```python
from build123d import *

# Parameters (mm, degrees)
ESQUISSE1_W             = 54.4
ESQUISSE1_H             = 15
BOSS_EXTRU_1_DEPTH      = 2
ESQUISSE2_W             = 2
ESQUISSE2_H             = 15
BOSS_EXTRU_2_DEPTH      = 35
CONG_1_R                = 1
ENL_V_MAT_EXTRU_1_REACH = 68.403
ESQUISSE3_R             = 1.6
ENL_V_MAT_EXTRU_2_REACH = 69.479
ESQUISSE4_R             = 1.6
ENL_V_MAT_EXTRU_3_REACH = 68.403
ESQUISSE6_R             = 1.5


with BuildPart() as part:
    # Esquisse1 → Boss.-Extru.1 (new body)
    with BuildSketch(Plane(origin=(0, 0, 0), x_dir=(1, 0, 0), z_dir=(0, 1, 0))):
        with Locations((27.2, 7.5)):
            Rectangle(ESQUISSE1_W, ESQUISSE1_H)
    extrude(amount=BOSS_EXTRU_1_DEPTH)

    # Esquisse2 → Boss.-Extru.2 (add)
    with BuildSketch(Plane.XZ):
        with Locations((1, -7.5)):
            Rectangle(ESQUISSE2_W, ESQUISSE2_H)
        with Locations((53.4, -7.5)):
            Rectangle(ESQUISSE2_W, ESQUISSE2_H)
    extrude(amount=BOSS_EXTRU_2_DEPTH)

    # Congé1
    cong_1_edges = [part.edges().sort_by_distance(p)[0] for p in [
        (52.4, 0, -7.5),
        (2, 0, -7.5),
    ]]
    fillet(cong_1_edges, radius=CONG_1_R)

    # Esquisse3 → Enlèv. mat.-Extru.1 (cut, up to next)
    with BuildSketch(Plane(origin=(54.4, 0, 0), x_dir=(0, 0, -1), z_dir=(1, 0, 0)), mode=Mode.PRIVATE) as enl_v_mat_extru_1_sk1:
        with Locations((7.5, -21.65)):
            Circle(ESQUISSE3_R)
    enl_v_mat_extru_1_tool1 = extrude(enl_v_mat_extru_1_sk1.sketch, amount=-ENL_V_MAT_EXTRU_1_REACH, mode=Mode.PRIVATE) & part.part
    add(enl_v_mat_extru_1_tool1.solids().sort_by_distance((54.4, -21.65, -7.5))[0], mode=Mode.SUBTRACT)

    # Esquisse4 → Enlèv. mat.-Extru.2 (cut, up to next)
    with BuildSketch(Plane(origin=(0, 2, 0), x_dir=(1, 0, 0), z_dir=(0, 1, 0)), mode=Mode.PRIVATE) as enl_v_mat_extru_2_sk1:
        with Locations(Location((42.4, 7.5, 0), (0, 0, 270))):
            Circle(ESQUISSE4_R)
    enl_v_mat_extru_2_tool1 = extrude(enl_v_mat_extru_2_sk1.sketch, amount=-ENL_V_MAT_EXTRU_2_REACH, mode=Mode.PRIVATE) & part.part
    # Esquisse4 → Enlèv. mat.-Extru.2 (cut, up to next)
    with BuildSketch(Plane(origin=(0, 2, 0), x_dir=(1, 0, 0), z_dir=(0, 1, 0)), mode=Mode.PRIVATE) as enl_v_mat_extru_2_sk2:
        with Locations(Location((6.4, 7.5, 0), (0, 0, 270))):
            Circle(ESQUISSE4_R)
    enl_v_mat_extru_2_tool2 = extrude(enl_v_mat_extru_2_sk2.sketch, amount=-ENL_V_MAT_EXTRU_2_REACH, mode=Mode.PRIVATE) & part.part
    # Esquisse4 → Enlèv. mat.-Extru.2 (cut, up to next)
    with BuildSketch(Plane(origin=(0, 2, 0), x_dir=(1, 0, 0), z_dir=(0, 1, 0)), mode=Mode.PRIVATE) as enl_v_mat_extru_2_sk3:
        with Locations(Location((24.4, 7.5, 0), (0, 0, 270))):
            Circle(ESQUISSE4_R)
    enl_v_mat_extru_2_tool3 = extrude(enl_v_mat_extru_2_sk3.sketch, amount=-ENL_V_MAT_EXTRU_2_REACH, mode=Mode.PRIVATE) & part.part
    add(enl_v_mat_extru_2_tool1.solids().sort_by_distance((42.4, 2, -7.5))[0], mode=Mode.SUBTRACT)
    add(enl_v_mat_extru_2_tool2.solids().sort_by_distance((6.4, 2, -7.5))[0], mode=Mode.SUBTRACT)
    add(enl_v_mat_extru_2_tool3.solids().sort_by_distance((24.4, 2, -7.5))[0], mode=Mode.SUBTRACT)

    # Esquisse6 → Enlèv. mat.-Extru.3 (cut, up to next)
    with BuildSketch(Plane.ZY, mode=Mode.PRIVATE) as enl_v_mat_extru_3_sk1:
        with Locations((-7.5, -13.86)):
            Circle(ESQUISSE6_R)
    enl_v_mat_extru_3_tool1 = extrude(enl_v_mat_extru_3_sk1.sketch, amount=-ENL_V_MAT_EXTRU_3_REACH, mode=Mode.PRIVATE) & part.part
    # Esquisse6 → Enlèv. mat.-Extru.3 (cut, up to next)
    with BuildSketch(Plane.ZY, mode=Mode.PRIVATE) as enl_v_mat_extru_3_sk2:
        with Locations((-7.5, -29.86)):
            Circle(ESQUISSE6_R)
    enl_v_mat_extru_3_tool2 = extrude(enl_v_mat_extru_3_sk2.sketch, amount=-ENL_V_MAT_EXTRU_3_REACH, mode=Mode.PRIVATE) & part.part
    add(enl_v_mat_extru_3_tool1.solids().sort_by_distance((0, -13.86, -7.5))[0], mode=Mode.SUBTRACT)
    add(enl_v_mat_extru_3_tool2.solids().sort_by_distance((0, -29.86, -7.5))[0], mode=Mode.SUBTRACT)


solid = part.part
```
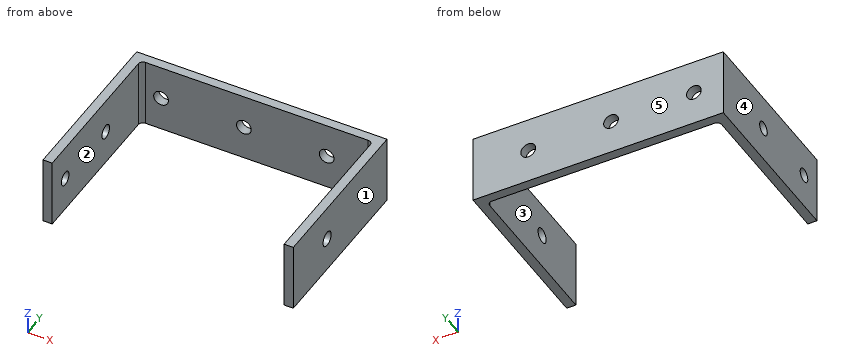
Model file for the job. Use its own axes, mm. Face numbers are marked on the shaded views. A direction names the side the tool comes from. Round coordinates to 2 decimals unless told otherwise and drop trailing zeros. Write each loop counter-clockwise with the first axis right and the second up, starting at its lowest first coordinate (ties: lowest second). Pieces come first, ordered by that corner, then holes. Notation, with made-up numbers: (-22, 43.25) - (-9, 43.25) arc R31 cw to (-9, 75.25) - close; hole circle Ø1 at (63.25, 9). An arc over 180 degrees is marked (long way). One line per item, written item: value.
(1) Cut at A-A, the plane x = 42.4. Give the cut face in (y, z).
Values follow:
outline: (0, -15) - (2, -15) - (2, -9.1) - (0, -9.1) - close; (0, -5.9) - (2, -5.9) - (2, 0) - (0, 0) - close
(2) Cut at C-C, the plane z = -7.5. Give the number of separate pieces and of enclosed holes in the cut face, plus the area to 3 significant figures.
Values follow:
separate pieces: 7
enclosed holes: 0
area: 212 mm²
(3) Wall check: probe 1 along Y at (x, z) = (0.75, -7.5); probe 2 along X at (y, z) = (0.7, -7.5); probe 3 along Y at (x, z) = (53.2, -7.5). Give the ranges that are in metal, low to high.
Values follow:
probe 1: y = -35 to -31.36, -28.36 to -15.36, -12.36 to 2
probe 2: x = 0 to 4.8, 8 to 22.8, 26 to 40.8, 44 to 54.4
probe 3: y = -35 to -23.25, -20.05 to 2
(4) Drop flat-ended pins along their axis: P1, Ø2.5, axis at x = 6.4, z = -7.5, coming from the +Y side; P2, Ø1.9, axis at y = -21.65, z = -7.5, coming from the +X side; P3, Ø5, axis at x = 29.5, z = -2, coming from the -Y side. Give the stop position or say it passes through.
Values follow:
P1: passes through
P2: stops at x = 2
P3: stops at y = 0
(5) Cut at D-D, the plane y = -4. Give the cut face in (x, z).
Values follow:
outline: (0, -15) - (2, -15) - (2, 0) - (0, 0) - close; (52.4, -15) - (54.4, -15) - (54.4, 0) - (52.4, 0) - close
(6) Two-plate mould, pull along X, no slides. Class the marked faces 3, 4 and 5: pulls with the +X half, pulls with the -X half, needs draft (parallel to the pull), parting line crosses it, or undercut.
Values follow:
face 3: undercut
face 4: pulls with the -X half
face 5: needs draft
(7) Cut at B-B, the plane y = -13.86. Give the cut face in (x, z), plus the area to 3 significant figures.
Values follow:
outline: (0, -15) - (2, -15) - (2, -9) - (0, -9) - close; (0, -6) - (2, -6) - (2, 0) - (0, 0) - close; (52.4, -15) - (54.4, -15) - (54.4, 0) - (52.4, 0) - close
area: 54.0 mm²
(8) 3-axis set-ups, long thin cutter, end or side, ignore diameter. For the marked faces 1 and 2: which of +Z, -Z, +X, -X, +Y, -Y reach the whole face in a straight line?
Values follow:
face 1: +Z, -Z, +X, +Y, -Y
face 2: +Z, -Z, -Y
